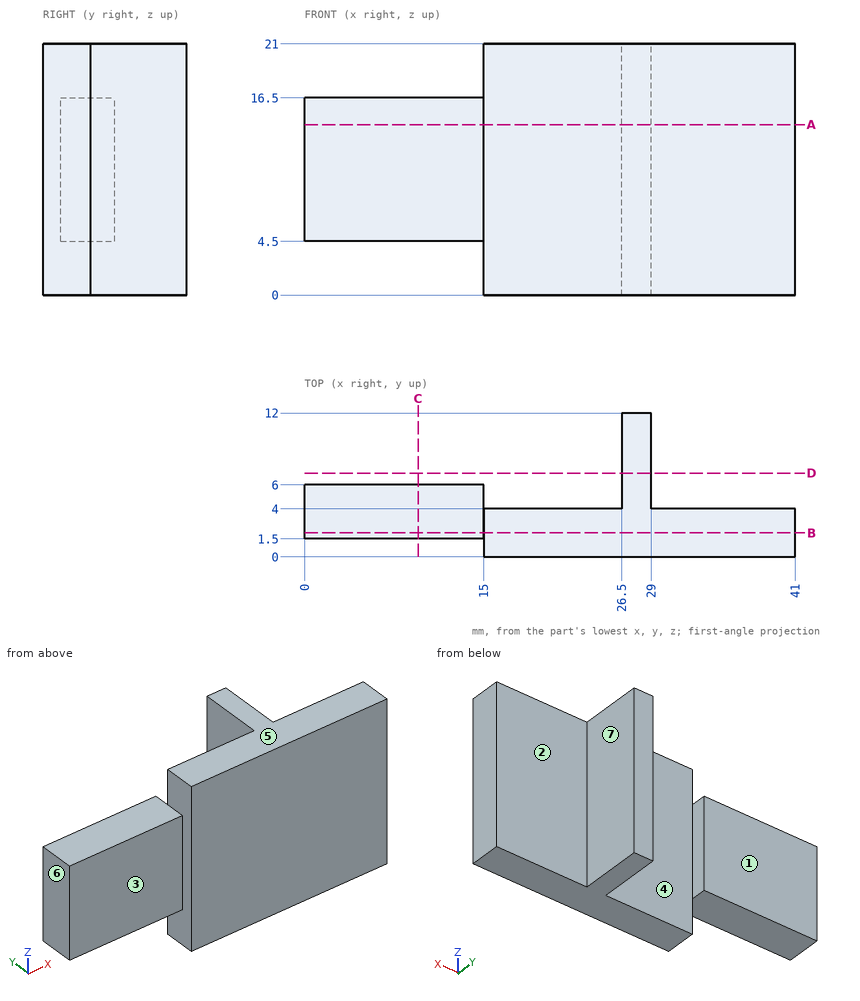
Geometry: see drawing. Coordinates: mm, zero at the bounding-box minimum. A direction names the side the tool comes from. Coordinates: 2 decimals unless noted, no trailing zeros. Loops run counter-clockwise (first coordinate to the right, second up) from the corner with the lowest first, then second, coordinate; pieces in that order, holes last.
Q1. Cut plane D-D (y = 7). Output: boundary loops of the cut face in (x, z).
Q2. Cut plane B-B (y = 2). Output: boundary loops of the cut face in (x, z), then the cut area to 3 significant figures.
Q3. Contact query for flat-ended pins moving along their axis: pin 1 (3.5 mm diameter, centred on x = 5.5, z = 9, fed in from -Y); pin 2 (3.5 mm diameter, centred on x = 10.5, y = 3.5, fed in from +Z); pin 3 (0.6 mm diameter, centred on y = 5.5, z = 12.5, fed in from +X). Output: stop coordinate, or through.
Q4. Draft query along X for the marked faces 4, 5, 6 and 7. Return one class per face: +X half, -X half, draft (parallel to the pull), parting line (faces both ways), or undercut.
Q5. Cut plane C-C (x = 9.5). Output: boundary loops of the cut face in (y, z), then the cut area to 3 significant figures.
Q6. Material intervals for line 1 (X direction, y = 5.25, z = 7.75); line 2 (X direction, y = 11.25, z = 4); line 3 (Y direction, x = 37, z = 5), sorted ascending.
Q7. Cut plane A-A (z = 14.25). Output: boundary loops of the cut face in (x, y), then the cut area to 4 significant figures.
Q8. Set-up query: the marked faces 1, 2 and 3. Return all of +Z, -Z, +X, -X, +Y, -Y with unobstructed straight access to the full face (end or side cutting, diameter ignored); none if empty.
Working result:
1. outline: (26.5, 0) - (29, 0) - (29, 21) - (26.5, 21) - close
2. outline: (0, 4.5) - (15, 4.5) - (15, 0) - (41, 0) - (41, 21) - (15, 21) - (15, 16.5) - (0, 16.5) - close
2. area: 726 mm2
3. pin 1: stops at y = 1.5
3. pin 2: stops at z = 16.5
3. pin 3: stops at x = 29
4. face 4: undercut
4. face 5: draft
4. face 6: -X half
4. face 7: +X half
5. outline: (1.5, 4.5) - (6, 4.5) - (6, 16.5) - (1.5, 16.5) - close
5. area: 54.0 mm2
6. line 1: x = 0 to 15, 26.5 to 29
6. line 2: x = 26.5 to 29
6. line 3: y = 0 to 4
7. outline: (0, 1.5) - (15, 1.5) - (15, 0) - (41, 0) - (41, 4) - (29, 4) - (29, 12) - (26.5, 12) - (26.5, 4) - (15, 4) - (15, 6) - (0, 6) - close
7. area: 191.5 mm2
8. face 1: +Z, -Z, -X, +Y
8. face 2: +Z, -Z, +X, +Y
8. face 3: +Z, -Z, -X, -Y
